Check sheet for the modelled part. Datum: model origin and axes. Units: mm. Face numbers are marked on the shaded views. A direction names the side the tool comes from. Give positions to 0.01 mm unless a question says otherwise; leave off trailing zeros. Order: outer loops, then holes, each group sorted by start corner. A loop starts at its lowest first (then second) coordinate and runs counter-clockwise, first axis right, second up. Notation, with made-up numbers: (19, 78) - (73, 78) arc R25 cw to (73, 111) - close; hole circle Ø2 at (31, 29). An arc over 180 degrees is marked (long way). Answer in a Markdown table with one row per item.
Autodesk Inventor part; units mm, degrees
ref_plane "工作平面1" through (0, 0, 5) normal (0, 0, 1) x (1, 0, 0)
ref_plane "YZ Plane" through (0, 0, 0) normal (1, 0, 0) x (0, 1, 0)
ref_plane "XZ Plane" through (0, 0, 0) normal (0, 1, 0) x (-1, 0, 0)
sketch "草圖1" plane through (0, 0, 0) normal (0, 0, 1) x (1, 0, 0)
  line L0 (0, 0) -> (5, 0)
  line L1 (5, 0) -> (5, 70)
  line L2 (5, 70) -> (0, 70)
  line L3 (0, 70) -> (0, 0)
  line L4 (0, 0) -> (12, 0)
  line L5 (12, 0) -> (12, 5)
  line L6 (12, 5) -> (0, 5)
  line L7 (0, 5) -> (0, 0)
  dimension "d0" = 10
  dimension "d1" = 70
  dimension "d2" = 5
  dimension "d3" = 12
revolve "迴轉1" add sketch "草圖1" angle 360 about axis through (0, 70, 0) along (0, -1, 0)
ref_plane "工作平面1" through (0, 0, 5) normal (0, 0, 1) x (1, 0, 0)
sketch "草圖2" plane through (0, 0, 5) normal (0, 0, 1) x (1, 0, 0)
  line L0 (-6, 0) -> (6, 0)
  line L1 (6, 0) -> (6, -12)
  line L2 (6, -12) -> (-6, -12)
  line L3 (-6, -12) -> (-6, 0)
  line L4 (-12, 0) -> (12, 0)
  circle A0 centre (0, -12) radius 6
  point P0 (0, 0)
  dimension "d6" = 12
  dimension "d7" = 12
extrude "擠出1" add sketch "草圖2" along normal blind 3
sketch "草圖3" plane through (0, 0, 8) normal (0, 0, 1) x (1, 0, 0)
  arc A0 (-6, -12) -> (6, -12) centre (0, -12) ccw
  circle A1 centre (0, -12) radius 2.5
  point P0 (0, 0)
  dimension "d10" = 5
extrude "擠出2" cut sketch "草圖3" against normal through all
mirror "鏡射1" about plane through (0, 0, 0) normal (0, 0, 1) of "擠出2", "擠出1"
properties part number "從動桿"
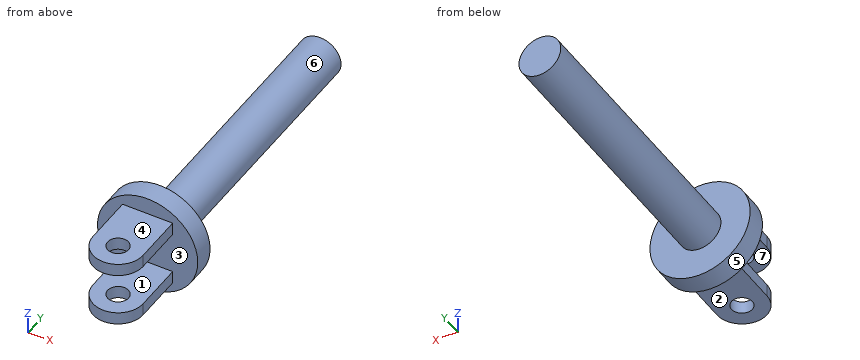
(1) Cross-section at A-A, the plane y = -1. Record the cut outline in (x, z).
Geometry says:
| item | result |
|---|---|
| outline | (-6, -8) - (6, -8) - (6, -5) - (-6, -5) - close; (-6, 5) - (6, 5) - (6, 8) - (-6, 8) - close |
(2) Access from +Z, -Z, +X, -X, +Y, -Y to the whole of each face (thin tool, end or side, straight path). Record for the marked faces 5, 6 and 7.
Geometry says:
| item | result |
|---|---|
| face 5 | +Y, -Y |
| face 6 | +Y |
| face 7 | +X, -X, -Y |
(3) Thickness scan on L1, parallel to Y at x = 0, z = 5.85; L2, parallel to X at y = -12, z = -6.3; L3, parallel to Y at x = 7, z = -5.75. Record the ranges inside material, lowest first.
Geometry says:
| item | result |
|---|---|
| L1 | -18 to -14.5, -9.5 to 5 |
| L2 | -6 to -2.5, 2.5 to 6 |
| L3 | 0 to 5 |
(4) Gauge pin test, flat ends, axial feed: P1, Ø10, axis at x = -7.5, z = -5.5, coming from the -Y side; P2, Ø1.5, axis at y = -3.5, z = -7, coming from the +X side; P3, Ø2.5, axis at y = -3, z = 6, coming from the -X side; P4, Ø3, axis at x = 0, y = -12, coming from the +Z side. Record the tip position at first contact, or that the pin passes through.
Geometry says:
| item | result |
|---|---|
| P1 | y = -17.45 |
| P2 | x = 6 |
| P3 | x = -6 |
| P4 | through |
(5) Cross-section at D-D, the plane z = -6.5. Record the cut outline in (x, y), then the cut area to 3 significant figures.
Geometry says:
| item | result |
|---|---|
| outline | (-10.09, 0) - (-6, 0) - (-6, -12) arc R6 ccw to (6, -12) - (6, 0) - (10.09, 0) - (10.09, 5) - (-10.09, 5) - close; hole circle Ø5 at (0, -12) |
| area | 282 mm² |
(6) Cross-section at B-B, the plane x = 0. Record the cut outline in (y, z), then the cut area to 3 significant figures.
Geometry says:
| item | result |
|---|---|
| outline | (-18, -8) - (-14.5, -8) - (-14.5, -5) - (-18, -5) - close; (-18, 5) - (-14.5, 5) - (-14.5, 8) - (-18, 8) - close; (-9.5, -8) - (0, -8) - (0, -12) - (5, -12) - (5, -5) - (70, -5) - (70, 5) - (5, 5) - (5, 12) - (0, 12) - (0, 8) - (-9.5, 8) - (-9.5, 5) - (0, 5) - (0, -5) - (-9.5, -5) - close |
| area | 848 mm² |
(7) Cross-section at C-C, the plane z = 0. Record the cut outline in (x, y).
Geometry says:
| item | result |
|---|---|
| outline | (-12, 0) - (12, 0) - (12, 5) - (5, 5) - (5, 70) - (-5, 70) - (-5, 5) - (-12, 5) - close |
(8) Mould release check, pull along Z, two halves, no side actions. Record for the marked faces 1, 2, 3 and 4: pulls with the +Z half, pulls with the -Z half, needs draft (parallel to the pull), parting line crosses it, or undercut.
Geometry says:
| item | result |
|---|---|
| face 1 | undercut |
| face 2 | pulls with the -Z half |
| face 3 | undercut |
| face 4 | pulls with the +Z half |
